Geometry check sheet. Reference: drawing and pictorial views, mm from the part's lowest x, y, z. A direction names the side the tool comes from. Round coordinates to 2 decimals unless told otherwise and drop trailing zeros. Write each loop counter-clockwise with the first axis right and the second up, starting at its lowest first coordinate (ties: lowest second). Pieces come first, ordered by that corner, then holes. Notation, with made-up numbers: M 48,-20 L 56,-20 A20 ccw 56,1 Z; hole C 73.5,67 d3. An arc over 180 degrees is marked long. One line per question, with ' | ' between items.
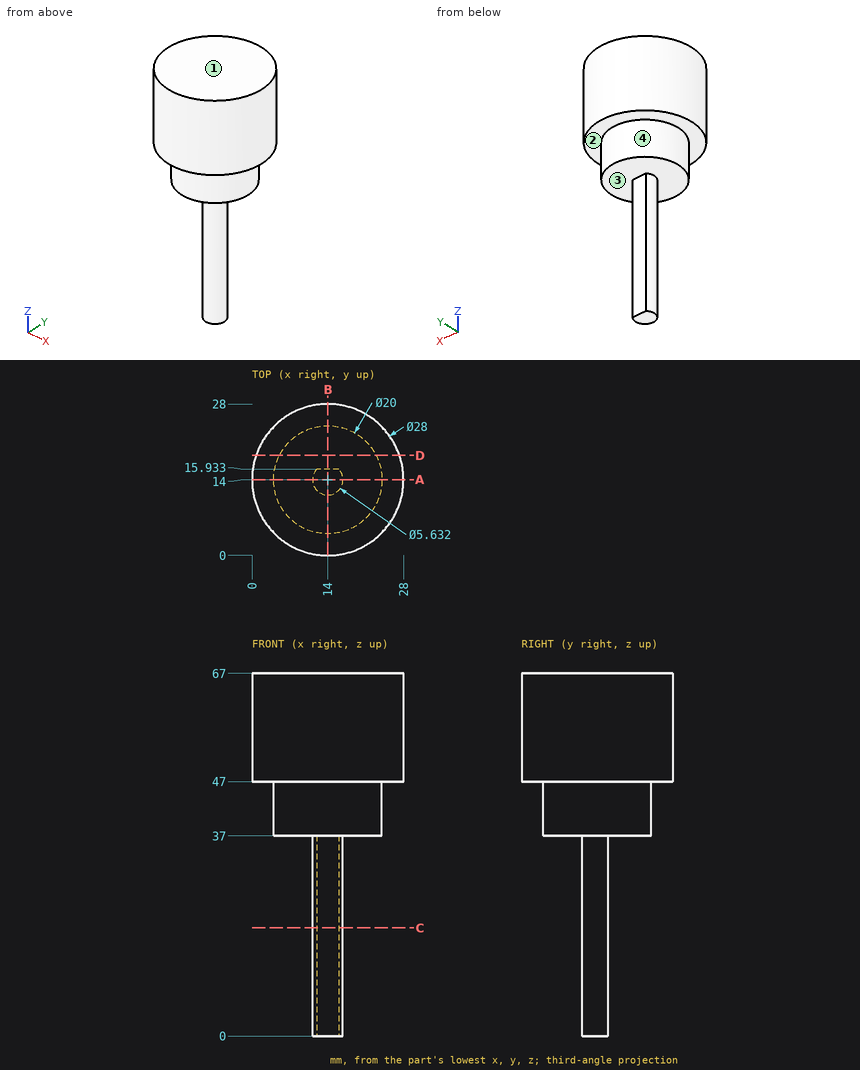
1. Go/stop test with flat-tipped pins: P1, Ø6, axis at y = 6.5, z = 8, coming from the +X side; P2, Ø6, axis at x = 13, z = 30.5, coming from the +Y side; P3, Ø4, axis at x = 21.5, z = 35.5, coming from the +Y side (1 decimal); P4, Ø6, axis at y = 7, z = 45.5, coming from the -X side. Record where each tip stops, or that it passes through.
Results:
P1: passes through | P2: stops at y = 15.93 | P3: stops at y = 21.9 | P4: stops at x = 0.71
2. Section check B-B, the plane x = 14. Record the cut outline in (y, z).
Results:
outline: M 0,47 L 4,47 L 4,37 L 11.18,37 L 11.18,0 L 15.93,0 L 15.93,37 L 24,37 L 24,47 L 28,47 L 28,67 L 0,67 Z
3. Tool access check on the marked faces 1 and 2. Record the directions out of +Z, -Z, +X, -X, +Y, -Y that give a thin tool (end or side, any length) a straight path to the whole face; none if there is none.
Results:
face 1: +Z, +X, -X, +Y, -Y | face 2: -Z
4. Mould release check, pull along Y, two halves, no side actions. Record for the marked faces 3 and 4: pulls with the +Y half, pulls with the -Y half, needs draft (parallel to the pull), parting line crosses it, or undercut.
Results:
face 3: needs draft | face 4: parting line crosses it
5. Section check D-D, the plane y = 18.5. Record the cut outline in (x, z), then the cut area to 3 significant figures.
Results:
outline: M 0.74,47 L 5.07,47 L 5.07,37 L 22.93,37 L 22.93,47 L 27.26,47 L 27.26,67 L 0.74,67 Z | area: 709 mm2
6. Section check A-A, the plane y = 14. Record the cut outline in (x, z).
Results:
outline: M 0,47 L 4,47 L 4,37 L 11.18,37 L 11.18,0 L 16.82,0 L 16.82,37 L 24,37 L 24,47 L 28,47 L 28,67 L 0,67 Z
7. Thickness scan on line 1 (Z direction, x = 10, y = 16.75); line 2 (Z direction, x = 25, y = 6); line 3 (Y direction, x = 18, z = 38.5) (1 decimal). Record the ranges inside material, lowest first.
Results:
line 1: z = 37 to 67 | line 2: z = 47 to 67 | line 3: y = 4.8 to 23.2
8. Section check C-C, the plane z = 20. Record the cut outline in (x, y), then the cut area to 3 significant figures.
Results:
outline: M 11.95,15.93 A2.82 ccw long 16.05,15.93 Z | area: 22.4 mm2
